```python
from build123d import *

# Parameters (mm, degrees)
BOSS_EXTRUDE1_DEPTH = 17.3
BOSS_EXTRUDE2_DEPTH = 3
CUT_EXTRUDE1_DEPTH  = 3
CUT_EXTRUDE2_DEPTH  = 1.7
FILLET1_DEPTH       = 17.3
FILLET1_START       = 6.212990815
FILLET1_2_DEPTH     = 2.287009185
FILLET1_3_DEPTH     = 2.287009085
FILLET1_START_2     = 3
FILLET1_4_DEPTH     = 8.5
FILLET2_R           = 1


with BuildPart() as part:
    # Sketch1 → Boss-Extrude1 (new body)
    with BuildSketch(Plane.XY):
        Polygon((6, 0), (7.5, 0), (7.5, 11.5), (-7.5, 11.5), (-7.5, 0), (-6, 0), (-6, 10), (6, 10), align=None)
    extrude(amount=BOSS_EXTRUDE1_DEPTH)

    # Sketch2 → Boss-Extrude2 (add)
    with BuildSketch(Plane.XZ):
        with BuildLine():
            Line((-7.5, 0), (-9.05, 0))
            ThreePointArc((-9.05, 0), (-13.3, 4.25), (-9.05, 8.5))
            Line((-9.05, 8.5), (-7.5, 8.5))
            Line((-7.5, 8.5), (-7.5, 0))
        make_face()
        with BuildLine():
            Line((7.5, 0), (9.05, 0))
            ThreePointArc((9.05, 0), (13.3, 4.25), (9.05, 8.5))
            Line((9.05, 8.5), (7.5, 8.5))
            Line((7.5, 8.5), (7.5, 0))
        make_face()
    extrude(amount=-BOSS_EXTRUDE2_DEPTH)

    # Sketch3 → Cut-Extrude1 (cut)
    with BuildSketch(Plane(origin=(0, 3, 0), x_dir=(1, 0, 0), z_dir=(0, 1, 0))):
        with BuildLine():
            Line((6, -2.95), (9, -2.95))
            ThreePointArc((9, -2.95), (10.3, -4.25), (9, -5.55))
            Line((9, -5.55), (6, -5.55))
            Line((6, -5.55), (6, -2.95))
        make_face()
        with BuildLine():
            Line((-6, -2.95), (-9, -2.95))
            ThreePointArc((-9, -2.95), (-10.3, -4.25), (-9, -5.55))
            Line((-9, -5.55), (-6, -5.55))
            Line((-6, -5.55), (-6, -2.95))
        make_face()
    extrude(amount=-CUT_EXTRUDE1_DEPTH, mode=Mode.SUBTRACT)

    # Sketch4 → Cut-Extrude2 (cut)
    with BuildSketch(Plane(origin=(0, 3, 0), x_dir=(1, 0, 0), z_dir=(0, 1, 0))):
        Polygon((9, -1.420983681), (7.5, -2.287009085), (6, -2.287009085), (6, -6.212990915), (7.5, -6.212990915), (9, -7.079016319), (11.45, -5.66450816), (11.45, -2.83549184), align=None)
        Polygon((-6, -6.212990915), (-7.5, -6.212990915), (-9, -7.079016319), (-11.45, -5.66450816), (-11.45, -2.83549184), (-9, -1.420983681), (-7.5, -2.287009085), (-6, -2.287009085), align=None)
    extrude(amount=-CUT_EXTRUDE2_DEPTH, mode=Mode.SUBTRACT)

    # Fillet1: read off the stored shape, not the designer's step
    # Fillet1 outline → Fillet1 (add)
    with BuildSketch(Plane.XY):
        with BuildLine():
            Line((6, 10), (3, 10))
            ThreePointArc((3, 10), (5.121320344, 9.121320344), (6, 7))
            Line((6, 7), (6, 10))
        make_face()
        with BuildLine():
            ThreePointArc((-6, 7), (-5.121320344, 9.121320344), (-3, 10))
            Line((-3, 10), (-6, 10))
            Line((-6, 10), (-6, 7))
        make_face()
    extrude(amount=FILLET1_DEPTH)

    # Fillet1 2 outline → Fillet1 2 (add)
    with BuildSketch(Plane.XY.offset(FILLET1_START)):
        with BuildLine():
            ThreePointArc((-7.5, 6), (-8.378679656, 3.878679656), (-10.5, 3))
            Line((-10.5, 3), (-7.5, 3))
            Line((-7.5, 3), (-7.5, 6))
        make_face()
        with BuildLine():
            ThreePointArc((10.5, 3), (8.378679656, 3.878679656), (7.5, 6))
            Line((7.5, 6), (7.5, 3))
            Line((7.5, 3), (10.5, 3))
        make_face()
    extrude(amount=FILLET1_2_DEPTH)

    # Fillet1 3 outline → Fillet1 3 (add)
    with BuildSketch(Plane.XY):
        with BuildLine():
            ThreePointArc((-7.5, 6), (-8.378679656, 3.878679656), (-10.5, 3))
            Line((-10.5, 3), (-7.5, 3))
            Line((-7.5, 3), (-7.5, 6))
        make_face()
        with BuildLine():
            ThreePointArc((10.5, 3), (8.378679656, 3.878679656), (7.5, 6))
            Line((7.5, 6), (7.5, 3))
            Line((7.5, 3), (10.5, 3))
        make_face()
    extrude(amount=FILLET1_3_DEPTH)

    # Fillet1 4 outline → Fillet1 4 (cut)
    with BuildSketch(Plane(origin=(0, 0, 0), x_dir=(1, 0, 0), z_dir=(0, 1, 0)).offset(FILLET1_START_2)):
        Polygon((9, -1.420983681), (7.5, -2.287009085), (10.5, -2.287009085), align=None)
        Polygon((10.5, -6.212990815), (7.5, -6.212990815), (9, -7.079016319), align=None)
        with BuildLine():
            Line((10.5, 0), (9.05, 0))
            ThreePointArc((9.05, 0), (9.786126109, -0.064236228), (10.5, -0.255003129))
            Line((10.5, -0.255003129), (10.5, 0))
        make_face()
        with BuildLine():
            ThreePointArc((10.5, -8.244996871), (9.786126109, -8.435763772), (9.05, -8.5))
            Line((9.05, -8.5), (10.5, -8.5))
            Line((10.5, -8.5), (10.5, -8.244996871))
        make_face()
        with BuildLine():
            Line((-9.05, 0), (-10.5, 0))
            Line((-10.5, 0), (-10.5, -0.255003129))
            ThreePointArc((-10.5, -0.255003129), (-9.786126109, -0.064236228), (-9.05, 0))
        make_face()
        with BuildLine():
            ThreePointArc((-9.05, -8.5), (-9.786126109, -8.435763772), (-10.5, -8.244996871))
            Line((-10.5, -8.244996871), (-10.5, -8.5))
            Line((-10.5, -8.5), (-9.05, -8.5))
        make_face()
        Polygon((-9, -1.420983681), (-10.5, -2.287009085), (-7.5, -2.287009085), align=None)
        Polygon((-7.5, -6.212990815), (-10.5, -6.212990815), (-9, -7.079016319), align=None)
    extrude(amount=FILLET1_4_DEPTH, mode=Mode.SUBTRACT)

    # Fillet2
    fillet2_edges = [part.edges().sort_by_distance(p)[0] for p in [
        (-7.5, 11.5, 8.65),
        (7.5, 11.5, 8.65),
    ]]
    fillet(fillet2_edges, radius=FILLET2_R)


solid = part.part
```
For this review, take the finished solid that the model builds, in its own axes (mm). A direction names the side the tool comes from. Coordinates: 2 decimals unless noted, no trailing zeros. Loops run counter-clockwise (first coordinate to the right, second up) from the corner with the lowest first, then second, coordinate; pieces in that order, holes last.
1. Insertion check: P1, Ø0.8, axis at x = 6.5, z = 4.5, coming from the -Y side; P2, Ø1.6, axis at x = -8.5, z = 5.5, coming from the +Y side; P3, Ø0.8, axis at x = 12.5, z = 4.5, coming from the +Y side. Each pin has a flat end and moves straight along its axis. Give the tip position at first contact, or say it passes through.
2. Add section A-A, the plane y = 2.25. Give the boundary of the cut face in (x, z), then the cut area to 3 significant figures.
3. For faces 1 (the flat face through (8, 1, 5.55)), 2 (the cylindrical face through (5.1, 9.14, 8.53)), 3 (the flat face through (12, 3, 4)), 4 (the flat face through (8, 3, 2)), list the 3-axis set-ups (+Z, -Z, +X, -X, +Y, -Y) from which the entire face can be reached by the end or side of a thin tool; tool diameter is ignored.
4. Add section C-C, the plane x = 8. Give the boundary of the cut face in (y, z), then the cut area to 3 significant figures.
5. Mouldability with a two-part tool opening along Y and no side actions: class faces 5 (the cylindrical face through (-8.36, 3.9, 0.87)), 6 (the flat face through (7, 3, 4)), 7 (the flat face through (-7, 2, 2.287)), 8 (the flat face through (-7.5, 6, 10)) as +Y half, -Y half, draft (parallel to the pull), parting line (faces both ways), or undercut.
6. Add section D-D, the plane y = 8.5. Give the boundary of the cut face in (x, z).
7. Add section B-B, the plane z = 4.25. Give the boundary of the cut face in (x, y), then the cut area to 3 significant figures.
8. For line 1 (X direction, y = 6.75, z = 16); line 2 (Y direction, x = -1.5, z = 6.5); line 3 (X direction, y = 9, z = 9), list the stretches that pass through material, from the lowest coordinate up.
Result:
1. P1: stops at y = 3
1. P2: stops at y = 1.3
1. P3: stops at y = 3
2. outline: (-11.45, 2.84) - (-11.45, 5.66) - (-9, 7.08) - (-7.5, 6.21) - (-6, 6.21) - (-6, 17.3) - (-7.5, 17.3) - (-7.5, 8.5) - (-9.05, 8.5) arc R4.25 ccw to (-9.05, 0) - (-6, 0) - (-6, 2.29) - (-7.5, 2.29) - (-9, 1.42) - close; (6, 0) - (9.05, 0) arc R4.25 ccw to (9.05, 8.5) - (7.5, 8.5) - (7.5, 17.3) - (6, 17.3) - (6, 6.21) - (7.5, 6.21) - (9, 7.08) - (11.45, 5.66) - (11.45, 2.84) - (9, 1.42) - (7.5, 2.29) - (6, 2.29) - close
2. area: 88.0 mm2
3. face 1: -Y
3. face 2: +Z, -Z, -Y
3. face 3: +Z, -Z, +X, +Y
3. face 4: +Y
4. outline: (0, 0) - (4.34, 0) - (4.34, 2) - (1.3, 2) - (1.3, 2.95) - (0, 2.95) - close; (0, 5.55) - (1.3, 5.55) - (1.3, 6.5) - (4.34, 6.5) - (4.34, 8.5) - (0, 8.5) - close
4. area: 19.8 mm2
5. face 5: +Y half
5. face 6: undercut
5. face 7: undercut
5. face 8: draft
6. outline: (-7.5, 0) - (-5.6, 0) - (-5.6, 17.3) - (-7.5, 17.3) - close; (5.6, 0) - (7.5, 0) - (7.5, 17.3) - (5.6, 17.3) - close
7. outline: (-13.3, 0) - (-10.3, 0) - (-10.3, 1.3) - (-11.45, 1.3) - (-11.45, 3) - (-13.3, 3) - close; (-7.5, 3) - (-6, 3) - (-6, 7) arc R3 cw to (-3, 10) - (3, 10) arc R3 cw to (6, 7) - (6, 3) - (7.5, 3) - (7.5, 10.5) arc R1 ccw to (6.5, 11.5) - (-6.5, 11.5) arc R1 ccw to (-7.5, 10.5) - close; (10.3, 0) - (13.3, 0) - (13.3, 3) - (11.45, 3) - (11.45, 1.3) - (10.3, 1.3) - close
7. area: 61.0 mm2
8. line 1: x = -7.5 to -6, 6 to 7.5
8. line 2: y = 10 to 11.5
8. line 3: x = -7.5 to -5.24, 5.24 to 7.5
